Design review of the part built by this model. Coordinates are the model's own, in mm. Face numbers are marked on the shaded views. Round coordinates to 2 decimals unless told otherwise and drop trailing zeros. Loops run counter-clockwise (first coordinate to the right, second up) from the corner with the lowest first, then second, coordinate; pieces in that order, holes last. Notation, with made-up numbers: (-2.75, -36) -> (52.25, -36) arc R22 ccw to (52.25, -13) -> close; hole circle Ø5 at (8.5, -2.75). An arc over 180 degrees is marked (long way). Answer as CSV lines item,"result". Start each with the question number.
(1) Draft analysis for pull direction Y (two halves, no side actions). For the marked faces 1, 2, 3 and 4, state which applies: +Y half, -Y half, draft (parallel to the pull), parting line (faces both ways), or undercut.
(2) To check wall thickness, follow line 1 (Y direction, x = -5.5, z = 7.5); line 2 (Y direction, x = -11.5, z = 5.25); line 3 (Y direction, x = 1, z = 21). State the ranges of each line that lie inside material, in increasing order. Write a range as from..to.
(3) Take a section at C-C, the plane z = 16.5. Write out the cut boundary in (x, y), and give its area (3 significant figures).
(4) Take a section at A-A, the plane x = 0. Write out the cut boundary in (y, z), and give its area (3 significant figures).
(5) Take a section at D-D, the plane x = 17. State how many separate pieces and enclosed holes the cut face has, and give its area (3 significant figures).
(6) For P1, Ø0.8, axis at x = -12, z = 29.5, coming from the -Y side; P2, Ø0.8, axis at y = -7.5, z = 29.5, coming from the +X side; P3, Ø1, axis at x = -13.5, z = 21.5, coming from the +Y side, all flat-tipped, find the tip position at first contact; note any pin that passes through.
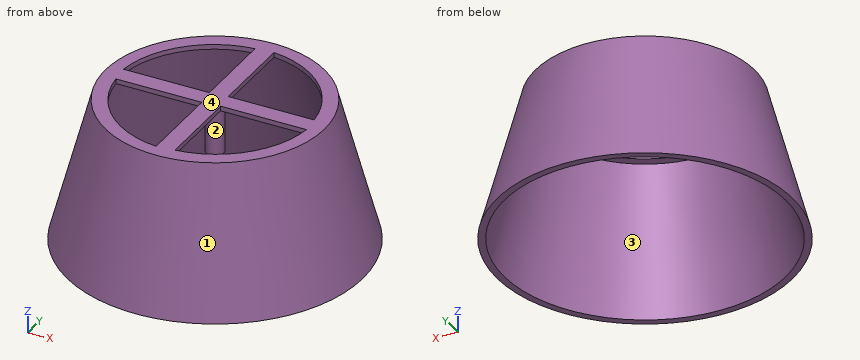
from build123d import *

# Parameters (mm, degrees)
F3_DEPTH = 25
F4_R     = 1.888711
F5_DEPTH = 10


with BuildPart() as f1:
    # F0 (on Front) → F1 (revolve)
    with BuildSketch(Plane.XZ):
        Polygon((21.7686, 28.996194), (29.538106, 0), (31.009124, 0), (22.970648, 30), (0, 30), (0, 28.996194), align=None)
    revolve(axis=Axis((0, 0, 15), (0, 0, -1)))

    # F2 (on face) → F3 (cut)
    with BuildSketch(Plane.XY.offset(30)):
        with BuildLine():
            Line((-2.089355, 1.671198), (-2.089355, 19.700249))
            ThreePointArc((-2.089355, 19.700249), (-14.319559, 13.901403), (-20.118406, 1.671198))
            Line((-20.118406, 1.671198), (-2.089355, 1.671198))
        make_face()
        with BuildLine():
            Line((1.671198, 20.118406), (1.671198, 2.089355))
            Line((1.671198, 2.089355), (19.700249, 2.089355))
            ThreePointArc((19.700249, 2.089355), (13.901403, 14.319559), (1.671198, 20.118406))
        make_face()
        with BuildLine():
            Line((-1.671198, -2.089355), (-19.700249, -2.089355))
            ThreePointArc((-19.700249, -2.089355), (-13.901403, -14.319559), (-1.671198, -20.118406))
            Line((-1.671198, -20.118406), (-1.671198, -2.089355))
        make_face()
        with BuildLine():
            Line((2.089355, -1.671198), (2.089355, -19.700249))
            ThreePointArc((2.089355, -19.700249), (14.319559, -13.901403), (20.118406, -1.671198))
            Line((20.118406, -1.671198), (2.089355, -1.671198))
        make_face()
    extrude(amount=-F3_DEPTH, mode=Mode.SUBTRACT)

    # F4 (on face) → F5 (join)
    with BuildSketch(Plane(origin=(0, 0, 28.996194), x_dir=(1, 0, 0), z_dir=(0, 0, -1))):
        Circle(F4_R)
    extrude(amount=F5_DEPTH)


solid = f1.part
The answers:
1,face 1,"parting line"
1,face 2,"undercut"
1,face 3,"undercut"
1,face 4,"draft"
2,line 1,"-28.47..-26.97, 26.97..28.47"
2,line 2,"-27.28..-25.67, 25.67..27.28"
2,line 3,"-25.36..-23.89, -1.6..1.6, 23.89..25.36"
3,outline,"circle Ø53.18 at (0, 0); hole circle Ø50.23 at (0, 0)"
3,area,"239 mm²"
4,outline,"(-31.01, 0) -> (-29.54, 0) -> (-21.77, 29) -> (-1.89, 29) -> (-1.89, 19) -> (1.89, 19) -> (1.89, 29) -> (21.77, 29) -> (29.54, 0) -> (31.01, 0) -> (22.97, 30) -> (-22.97, 30) -> close"
4,area,"169 mm²"
5,separate pieces,"3"
5,enclosed holes,"0"
5,area,"127 mm²"
6,P1,"y = -20.01"
6,P2,"x = 22.03"
6,P3,"y = 21.68"
